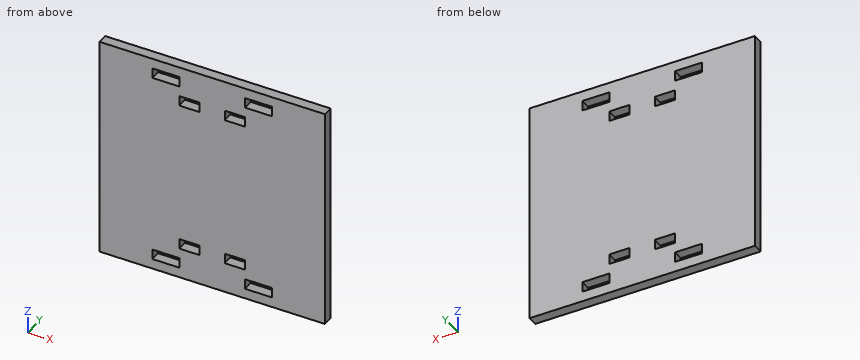
from build123d import *

# Parameters (mm, degrees)
ESBO_O1_W                = 6
ESBO_O1_H                = 3
RESSALTO_EXTRUS_O1_DEPTH = 3


with BuildPart() as part:
    # Esboço1 → Ressalto-extrusão1 (new body)
    with BuildSketch(Plane(origin=(0, 0, 0), x_dir=(1, 0, 0), z_dir=(0, 1, 0))):
        Polygon((-33.5, 28), (-33.5, -27.5), (-33.5, -28), (-33.5, -33), (-9.75, -33), (33.5, -33), (33.5, -28), (33.5, -27.5), (33.5, 28), (33.5, 33), (-9.75, 33), (-33.5, 33), align=None)
        Polygon((-16.929303449, -27), (-9.75, -27), (-9.75, -28.5), (-9.75, -30), (-17.75, -30), (-17.75, -27), align=None, mode=Mode.SUBTRACT)
        with Locations((-6.75, -22.5)):
            Rectangle(ESBO_O1_W, ESBO_O1_H, mode=Mode.SUBTRACT)
        Polygon((9.75, -28.5), (9.75, -27), (17.75, -27), (17.75, -30), (9.75, -30), align=None, mode=Mode.SUBTRACT)
        with Locations((6.75, -22.5)):
            Rectangle(ESBO_O1_W, ESBO_O1_H, mode=Mode.SUBTRACT)
        with Locations((-6.75, 22.5)):
            Rectangle(ESBO_O1_W, ESBO_O1_H, mode=Mode.SUBTRACT)
        Polygon((-9.75, 28.5), (-9.75, 27), (-16.929303449, 27), (-17.75, 27), (-17.75, 30), (-9.75, 30), align=None, mode=Mode.SUBTRACT)
        with Locations((6.75, 22.5)):
            Rectangle(ESBO_O1_W, ESBO_O1_H, mode=Mode.SUBTRACT)
        Polygon((9.75, 27), (9.75, 28.5), (9.75, 30), (17.75, 30), (17.75, 27), align=None, mode=Mode.SUBTRACT)
    extrude(amount=RESSALTO_EXTRUS_O1_DEPTH)


solid = part.part
Work out the finished part from the listing and answer in its coordinate system (mm). Give positions to 0.01 mm unless a question says otherwise; leave off trailing zeros. Write each loop counter-clockwise with the first axis right and the second up, starting at its lowest first coordinate (ties: lowest second). Pieces come first, ordered by that corner, then holes. Notation, with made-up numbers: (64, 80.5) - (105, 80.5) arc R24 ccw to (105, 119.5) - close; hole circle Ø7 at (5, 49). An arc over 180 degrees is marked (long way). One line per item, written item: value. Start each with the question number.
1. Find section B-B (z = -23). Write down the section's boundary in (x, y), then the cut area to 3 significant figures.
2. Find section A-A (x = -12). Write down the section's boundary in (y, z).
3. Find section C-C (y = 2.05). State how many separate pieces and enclosed holes the cut face has, then the cut area to 3 significant figures.
4. Consider probe 1 along Z at (x, y) = (-7.5, 2.6); probe 2 along Z at (x, y) = (14.5, 2.7); probe 3 along X at (y, z) = (2.15, -28). Determine where each line is inside the solid, lowest interval first.
Geometry results:
1. outline: (-33.5, 0) - (-9.75, 0) - (-9.75, 3) - (-33.5, 3) - close; (-3.75, 0) - (3.75, 0) - (3.75, 3) - (-3.75, 3) - close; (9.75, 0) - (33.5, 0) - (33.5, 3) - (9.75, 3) - close
1. area: 165 mm2
2. outline: (0, -33) - (3, -33) - (3, -30) - (0, -30) - close; (0, -27) - (3, -27) - (3, 27) - (0, 27) - close; (0, 30) - (3, 30) - (3, 33) - (0, 33) - close
3. separate pieces: 1
3. enclosed holes: 8
3. area: 4,250 mm2
4. probe 1: -33 to -24, -21 to 21, 24 to 33
4. probe 2: -33 to -30, -27 to 27, 30 to 33
4. probe 3: -33.5 to -17.75, -9.75 to 9.75, 17.75 to 33.5
